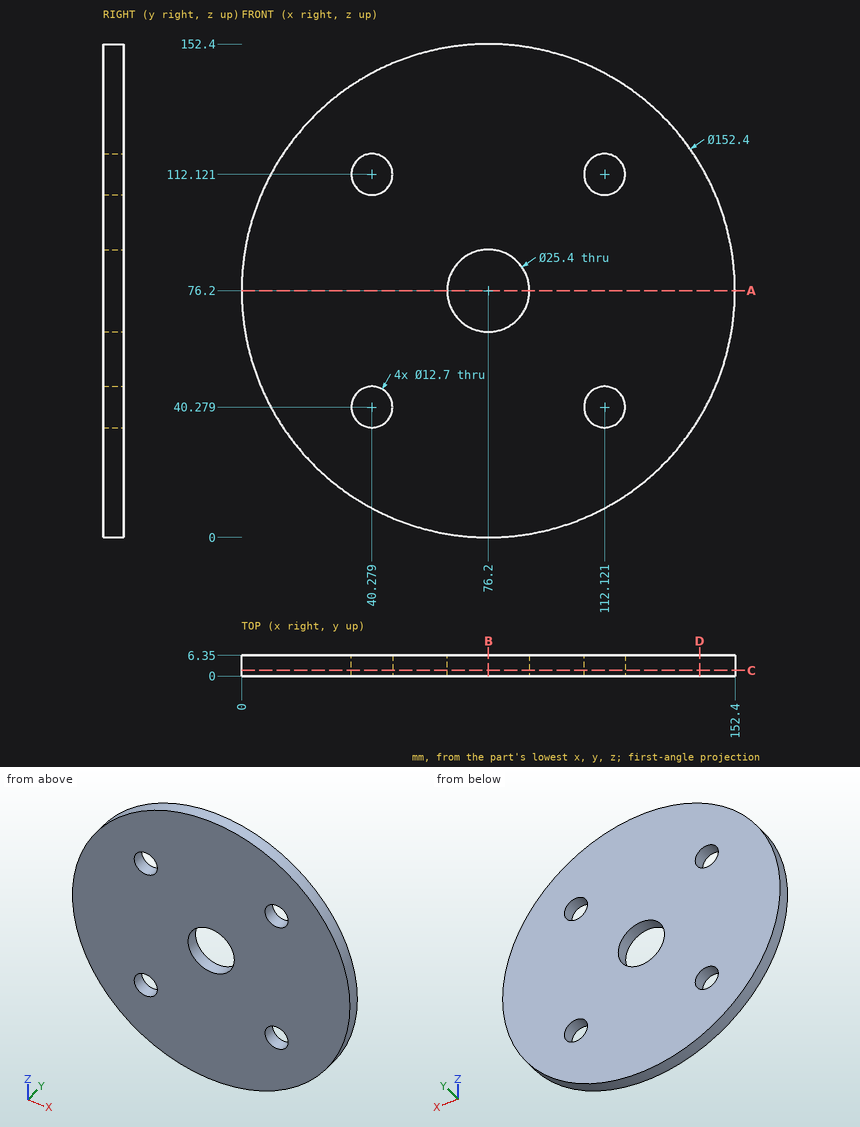
Print and shaded views of the part. All mm, measured from the part's lowest x, y and z. Give positions to 0.01 mm unless a question says otherwise; leave off trailing zeros. Write each loop counter-clockwise with the first axis right and the second up, starting at its lowest first coordinate (ties: lowest second). Pieces come first, ordered by that corner, then holes. Notation, with made-up numbers: (89.5, -33) - (146.5, -33) arc R30 cw to (146.5, 0) - close; hole circle Ø8 at (10, 23). An arc over 180 degrees is marked (long way). Put each result on its own line as item: value.
(1) Saw through at C-C (y = 1.75). List the corners of the cut face in (x, z), then the cut area to 3 significant figures.
Working result:
outline: circle Ø152.4 at (76.2, 76.2); hole circle Ø12.7 at (40.28, 40.28); hole circle Ø12.7 at (40.28, 112.12); hole circle Ø25.4 at (76.2, 76.2); hole circle Ø12.7 at (112.12, 40.28); hole circle Ø12.7 at (112.12, 112.12)
area: 17,200 mm^2
(2) Saw through at D-D (x = 141.5). List the corners of the cut face in (y, z), then the cut area to 3 significant figures.
Working result:
outline: (0, 36.93) - (6.35, 36.93) - (6.35, 115.47) - (0, 115.47) - close
area: 499 mm^2
(3) Drop a flat-ended pin along its axis: pin 1 Ø10 at (x, z) = (40.28, 112.12) entering from -Y (1 decimal). Give the stop position or say it passes through.
Working result:
pin 1: through
(4) Saw through at A-A (z = 76.2). List the corners of the cut face in (x, y).
Working result:
outline: (0, 0) - (63.5, 0) - (63.5, 6.35) - (0, 6.35) - close; (88.9, 0) - (152.4, 0) - (152.4, 6.35) - (88.9, 6.35) - close
(5) Wall check: L1, parallel to Z at x = 115, y = 2.25; L2, parallel to X at y = 4.5, z = 116; L3, parallel to X at y = 4.5, z = 85.5. Give the ranges that are in metal, low to high.
Working result:
L1: 10.62 to 34.62, 45.94 to 106.46, 117.78 to 141.78
L2: 11.22 to 35.25, 45.31 to 107.09, 117.15 to 141.18
L3: 0.57 to 67.55, 84.85 to 151.83
(6) Saw through at B-B (x = 76.2). List the corners of the cut face in (y, z), then the cut area to 3 significant figures.
Working result:
outline: (0, 0) - (6.35, 0) - (6.35, 63.5) - (0, 63.5) - close; (0, 88.9) - (6.35, 88.9) - (6.35, 152.4) - (0, 152.4) - close
area: 806 mm^2
